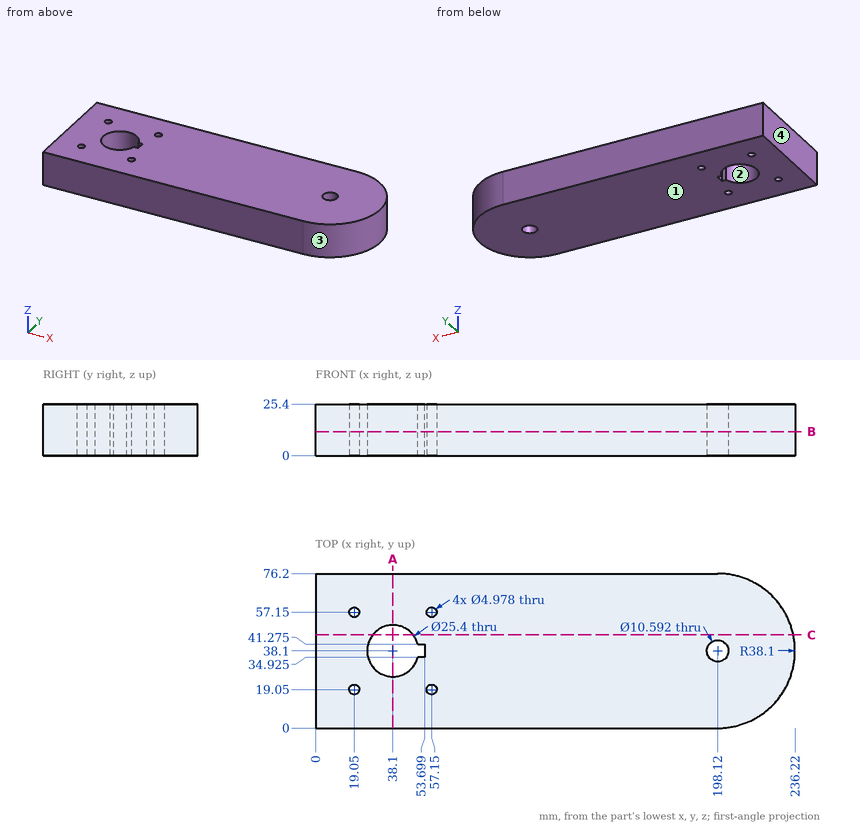
Answer from the drawing. Dimensions are ordinates in mm from the lowest x, y and z of the part. Coordinates: 2 decimals unless noted, no trailing zeros. Write each loop counter-clockwise with the first axis right and the second up, starting at its lowest first coordinate (ties: lowest second). Pieces come first, ordered by that corner, then holes. Notation, with made-up numbers: (-31, 88) - (-14, 88) arc R13 cw to (-14, 96) - close; hole circle Ø9 at (63.5, 85.5). An arc over 180 degrees is marked (long way). Return JSON: item names as keys, results as strings. Group by question number.
Q1. The part is cut by section A-A on x = 38.1. Write down the section's boundary in (y, z).
Q2. Find the intervals of material crossed by line 1 along X through (y, z) = (19.05, 5.5) (1 decimal); line 2 along X through (y, z) = (38.5, 18.5); line 3 along Y through (x, z) = (198, 18.5) (1 decimal), in increasing order. Write a range as [from, to].
Q3. Flat-ended cylindrical pins translate along their axes: pin 1 Ø12 at (x, y) = (131.5, 42.5) entering from -Z; pin 2 Ø4 at (x, y) = (57.15, 19.05) entering from +Z. Find the tip coordinate at first contact, or state that the pin passes through.
Q4. The part is cut by section B-B on z = 11.75. State how many separate pieces and enclosed holes the cut face has, and give its area (3 significant figures).
Q5. For a pull along X with two mould halves and no side action, classify the marked faces 1, 2, 3 and 4 as +X half, -X half, draft (parallel to the pull), parting line (faces both ways), or undercut.
Q6. The part is cut by section C-C on y = 46. Write down the section's boundary in (x, z), and give its area (3 significant figures).
Evaluation:
{
 "1": {"outline": "(0, 0) - (25.4, 0) - (25.4, 25.4) - (0, 25.4) - close; (50.8, 0) - (76.2, 0) - (76.2, 25.4) - (50.8, 25.4) - close"},
 "2": {"line 1": "x = [0, 16.6], [21.5, 54.7], [59.6, 231.1]", "line 2": "x = [0, 25.41], [53.7, 192.84], [203.4, 236.22]", "line 3": "y = [0, 32.8], [43.4, 76.2]"},
 "3": {"pin 1": "stops at z = 0", "pin 2": "passes through"},
 "4": {"separate pieces": "1", "enclosed holes": "6", "area": "16,700 mm2"},
 "5": {"face 1": "draft", "face 2": "undercut", "face 3": "+X half", "face 4": "-X half"},
 "6": {"outline": "(0, 0) - (28.16, 0) - (28.16, 25.4) - (0, 25.4) - close; (48.04, 0) - (235.39, 0) - (235.39, 25.4) - (48.04, 25.4) - close", "area": "5,470 mm2"}
}
